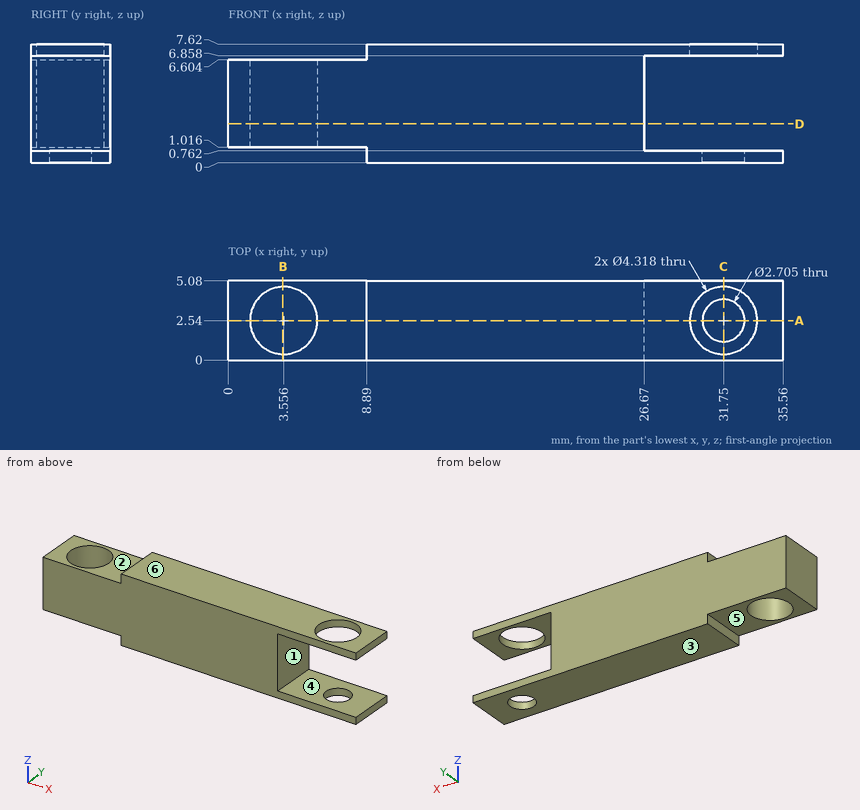
For this review, use the dimensioned drawing (mm, ordinates from the lowest corner) and the shaded views. A direction names the side the tool comes from. Coordinates: 2 decimals unless noted, no trailing zeros. Write each loop counter-clockwise with the first axis right and the second up, starting at its lowest first coordinate (ties: lowest second). Pieces come first, ordered by that corner, then holes. Notation, with made-up numbers: (2, 3) - (17, 3) arc R29 cw to (17, 32) - close; hole circle Ø2 at (-8, 2). An arc over 180 degrees is marked (long way). Answer in a Markdown table with one row per item. Add a question column.
Q1. To check wall thickness, follow line 1 along Z through (x, y) = (28, 2.5); line 2 along Z through (x, y) = (33, 1.6); line 3 along Z through (x, y) = (8.5, 4.2). State the ranges of each line that lie inside material, in increasing order. Write a range as from..to.
Q2. Consider section D-D on z = 2.5. Give the boundary of the cut face in (x, y) (3 decimals), then the cut area to 3 significant figures.
Q3. Consider section C-C on x = 31.75. Give the boundary of the cut face in (y, z).
Q4. Clearance check with flat-ended pins moving along their axes: pin 1 (2.5 mm diameter, centred on y = 3, z = 5, fed in from +X); pin 2 (0.5 mm diameter, centred on y = 3, z = 0.5, fed in from -X); pin 3 (2.5 mm diameter, centred on x = 2.5, y = 2, fed in from +Z). State where each tip first meets the part, or that it passes through.
Q5. For the marked faces 1, 2 and 3, list the 3-axis set-ups (+Z, -Z, +X, -X, +Y, -Y) from which the entire face can be reached by the end or side of a thin tool; tool diameter is ignored.
Q6. Draft analysis for pull direction Z (two halves, no side actions). For the marked faces 4, 5 and 6, state which applies: +Z half, -Z half, draft (parallel to the pull), parting line (faces both ways), or undercut.
Q7. Consider section B-B on x = 3.5. Give the boundary of the cut face in (y, z).
Q8. Consider section A-A on y = 2.54. Give the boundary of the cut face in (x, z) (1 decimal), then the cut area to 3 significant figures.
Answers below:
| question | item | result |
|---|---|---|
| 1 | line 1 | 0..0.76, 6.86..7.62 |
| 1 | line 2 | 0..0.76 |
| 1 | line 3 | 1.02..6.6 |
| 2 | outline | (0, 0) - (26.67, 0) - (26.67, 5.08) - (0, 5.08) - close; hole circle Ø4.318 at (3.556, 2.54) |
| 2 | area | 121 mm² |
| 3 | outline | (0, 0) - (1.19, 0) - (1.19, 0.76) - (0, 0.76) - close; (0, 6.86) - (0.38, 6.86) - (0.38, 7.62) - (0, 7.62) - close; (3.89, 0) - (5.08, 0) - (5.08, 0.76) - (3.89, 0.76) - close; (4.7, 6.86) - (5.08, 6.86) - (5.08, 7.62) - (4.7, 7.62) - close |
| 4 | pin 1 | x = 26.67 |
| 4 | pin 2 | x = 8.89 |
| 4 | pin 3 | z = 6.6 |
| 5 | face 1 | +X, +Y, -Y |
| 5 | face 2 | +Z, -X, +Y, -Y |
| 5 | face 3 | -Z, +X, -X, +Y, -Y |
| 6 | face 4 | undercut |
| 6 | face 5 | -Z half |
| 6 | face 6 | +Z half |
| 7 | outline | (0, 1.02) - (0.38, 1.02) - (0.38, 6.6) - (0, 6.6) - close; (4.7, 1.02) - (5.08, 1.02) - (5.08, 6.6) - (4.7, 6.6) - close |
| 8 | outline | (0, 1) - (1.4, 1) - (1.4, 6.6) - (0, 6.6) - close; (5.7, 1) - (8.9, 1) - (8.9, 0) - (30.4, 0) - (30.4, 0.8) - (26.7, 0.8) - (26.7, 6.9) - (29.6, 6.9) - (29.6, 7.6) - (8.9, 7.6) - (8.9, 6.6) - (5.7, 6.6) - close; (33.1, 0) - (35.6, 0) - (35.6, 0.8) - (33.1, 0.8) - close; (33.9, 6.9) - (35.6, 6.9) - (35.6, 7.6) - (33.9, 7.6) - close |
| 8 | area | 169 mm² |
